Autodesk Fusion 360 part; units mm, degrees
sketch "Sketch1" plane through (0, 0, 0) normal (1, 0, 0) x (0, 1, 0)
  line L0 (0, 0) -> (11, 0) construction
  line L1 (0, 0) -> (60, 0)
  line L2 (60, 0) -> (60, 5)
  line L3 (60, 5) -> (41, 5) construction
  line L4 (0, 5) -> (0, 0) construction
  line L5 (0, 0) -> (0, 9)
  line L6 (11, 0) -> (11, 30) construction
  line L7 (0, 9) -> (11, 9)
  line L8 (11, 9) -> (11, 30)
  line L9 (11, 30) -> (17, 30)
  line L10 (17, 30) -> (17, 29)
  arc A0 (17, 29) -> (41, 5) centre (41, 29) ccw
  line L11 (41, 5) -> (60, 5)
  dimension "d1" = 11
  dimension "d2" = 60
  dimension "d3" = 5
  dimension "d4" = 9
  dimension "d5" = 30
  dimension "d6" = 6
  dimension "d7" = 24
revolve "Revolve1" add sketch "Sketch1" angle 360 about axis through (0, 0, 5) along (0, 0, -1)
sketch "Sketch2" plane through (0, 0, 5) normal (0, 0, 1) x (-1, 0, 0)
  circle A0 centre (0, 0) radius 41
  circle A1 centre (0, 0) radius 60
  line L0 (0, 0) -> (0, 35) construction
  line L1 (0, 0) -> (-35, 0) construction
  line L2 (-35, 0) -> (-35, 35) construction
  line L3 (-35, 35) -> (0, 35) construction
  circle A2 centre (-35, 35) radius 2
  circle A3 centre (-35, -35) radius 2
  circle A4 centre (35, -35) radius 2
  circle A5 centre (35, 35) radius 2
  dimension "d9" = 35
  dimension "d10" = 35
  dimension "d11" = 4
  dimension "d13" = 360
extrude "Extrude2" cut sketch "Sketch2" against normal blind 6 contours A2 | A3 | A4 | A5
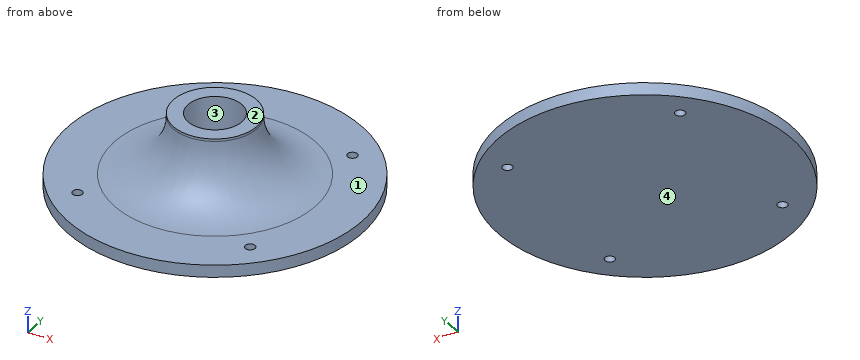
Source: CAD feature listing. Evaluate the final solid. Frame: model axes, mm. Face numbers are marked on the shaded views. A direction names the side the tool comes from. Round coordinates to 2 decimals unless told otherwise and drop trailing zeros. Write each loop counter-clockwise with the first axis right and the second up, starting at its lowest first coordinate (ties: lowest second). Pieces come first, ordered by that corner, then holes. Notation, with made-up numbers: M -34.5,-23 L 20.5,-23 A17 cw 20.5,6 Z; hole C 44.25,-18 d8. An arc over 180 degrees is marked long. Answer as a JSON object with one key per item and string values. Group by question number.
(1) Mould query, pull axis X, two halves, no side actions, for the marked faces 3 and 4. Classes: +X half, -X half, draft (parallel to the pull), parting line (faces both ways), or undercut.
(2) Reachability of the marked faces 1 and 2 from +Z, -Z, +X, -X, +Y, -Y: full face, straight path, thin tool, end or side. Return the list, or none.
(3) Section query A-A on y = 0. Output: boundary loops of the cut face in (x, z), then the cut area to 3 significant figures.
(4) Section query D-D on z = 25. Output: boundary loops of the cut face in (x, y).
(5) First-contact query: pin 1 (1 mm diameter, centred on y = 4, z = 18.5, fed in from +X); pin 2 (4 mm diameter, centred on x = -37, y = 9.5, fed in from +Z); pin 3 (1.5 mm diameter, centred on x = -6, z = 4.5, fed in from +Y); pin 4 (3 mm diameter, centred on x = 35, y = -35, fed in from +Z). Flat tips, straight axial feed; report the tip coordinate or a pass-through.
(6) Ray query, line 1 (X direction, y = -35, z = 1.55); line 2 (Z direction, x = -3, y = 50.5). Return the intervals inside material, ascending. Write a range as [from, to].
(7) Section query C-C on y = -35. State how many separate pieces and enclosed holes the cut face has, then the cut area to 3 significant figures.
Computed values:
{
 "1": {"face 3": "undercut", "face 4": "draft"},
 "2": {"face 1": "+Z", "face 2": "+Z, +X, -X, +Y, -Y"},
 "3": {"outline": "M -60,0 L 60,0 L 60,5 L 41,5 A24 cw 17,29 L 17,30 L 11,30 L 11,9 L -11,9 L -11,30 L -17,30 L -17,29 A24 cw -41,5 L -60,5 Z", "area": "1,240 mm^2"},
 "4": {"outline": "C 0,0 d34.67; hole C 0,0 d22"},
 "5": {"pin 1": "x = 19.28", "pin 2": "z = 5.48", "pin 3": "y = 59.77", "pin 4": "through"},
 "6": {"line 1": "[-48.73, -37], [-33, 33], [37, 48.73]", "line 2": "[0, 5]"},
 "7": {"separate pieces": "3", "enclosed holes": "0", "area": "464 mm^2"}
}
